```python
from build123d import *

# Parameters (mm, degrees)
BOSS_EXTRU_1_DEPTH = 3


with BuildPart() as part:
    # Esquisse1 → Boss.-Extru.1 (new body)
    with BuildSketch(Plane(origin=(0, 0, 0), x_dir=(1, 0, 0), z_dir=(0, 1, 0))):
        Polygon((3, 31.833333333), (0, 31.833333333), (0, 23.166666667), (3, 23.166666667), (3, 17.466666667), (3, 11.766666667), (0, 11.766666667), (0, 3.1), (3, 3.1), (3, 3), (5.7, 3), (5.7, 0), (14.3, 0), (14.3, 3), (25.7, 3), (25.7, 0), (34.3, 0), (34.3, 3), (45.7, 3), (45.7, 0), (54.3, 0), (54.3, 3), (65.7, 3), (65.7, 0), (74.3, 0), (74.3, 3), (85.7, 3), (85.7, 0), (94.3, 0), (94.3, 3), (97, 3), (97, 3.1), (100, 3.1), (100, 11.766666667), (97, 11.766666667), (97, 23.166666667), (100, 23.166666667), (100, 31.833333333), (97, 31.833333333), (97, 43.233333333), (100, 43.233333333), (100, 51.9), (97, 51.9), (97, 52), (94.3, 52), (94.3, 55), (85.7, 55), (85.7, 52), (74.3, 52), (74.3, 55), (65.7, 55), (65.7, 52), (54.3, 52), (54.3, 55), (45.7, 55), (45.7, 52), (34.3, 52), (34.3, 55), (25.7, 55), (25.7, 52), (20, 52), (14.3, 52), (14.3, 55), (5.7, 55), (5.7, 52), (3, 52), (3, 51.9), (0, 51.9), (0, 43.233333333), (3, 43.233333333), align=None)
    extrude(amount=BOSS_EXTRU_1_DEPTH)


solid = part.part
```
Could you check a few things on this model? Use its own coordinates, in mm. A direction names the side the tool comes from. Round coordinates to 2 decimals unless told otherwise and drop trailing zeros. Loops run counter-clockwise (first coordinate to the right, second up) from the corner with the lowest first, then second, coordinate; pieces in that order, holes last. Notation, with made-up numbers: M 49,-26.75 L 57,-26.75 A24 cw 57,8.25 Z; hole C 75,-15.75 d1. An arc over 180 degrees is marked long. Answer as CSV lines item,"result".
1) Which directions (+Z, -Z, +X, -X, +Y, -Y) give clear straight access to the entire face, cutting with the end or side of a thin tool? Please do faces 1 (the flat face through (1, 1, -43.233)), 2 (the flat face through (99, 1, -11.767)), 3 (the flat face through (1, 1, -3.1)).
From the geometry:
face 1,"-X, +Y, -Y"
face 2,"+X, +Y, -Y"
face 3,"+Z, -X, +Y, -Y"
2) If I drill on probe 1 along Z at (x, y) = (63, 2.85); probe 2 along X at (y, z) = (1.75, -36.5), over which ranges is the centre line in solid material (lowest first)?
From the geometry:
probe 1,"-52 to -3"
probe 2,"3 to 97"
3) Imagine slicing it at B-B on z = -20.5. List the corners of the cut face in (x, y) for me, and give its area (3 significant figures).
From the geometry:
outline,"M 3,0 L 97,0 L 97,3 L 3,3 Z"
area,"282 mm^2"
4) For pin 1 Ø0.9 at (y, z) = (1, -2) entering from -X; pin 2 Ø1.5 at (y, z) = (1.5, -1.5) entering from +X; pin 3 Ø0.9 at (y, z) = (1, -15) entering from +X, each with a flat end and sliding along its axis, tell me the tip position at first contact or that it passes through.
From the geometry:
pin 1,"x = 5.7"
pin 2,"x = 94.3"
pin 3,"x = 97"
5) Imagine slicing it at A-A on x = 18. List the corners of the cut face in (y, z) for me, and give its area (3 significant figures).
From the geometry:
outline,"M 0,-52 L 3,-52 L 3,-3 L 0,-3 Z"
area,"147 mm^2"
6) We'd pull the mould along X, two halves only. Please class faces 4 (the flat face through (70, 1, -55)), 5 (the flat face through (5.7, 1, -54)), 6 (the flat face through (65.7, 1, -2)): released by +X, released by -X, zero draft, split by the parting line, or undercut.
From the geometry:
face 4,"zero draft"
face 5,"released by -X"
face 6,"undercut"
